```python
from build123d import *

# Parameters (mm, degrees)
SKETCH1_W           = 14
SKETCH1_H           = 80
BOSS_EXTRUDE1_DEPTH = 2
SKETCH2_W           = 14
SKETCH2_H           = 80
SKETCH2_W_2         = 10
SKETCH2_H_2         = 75
BOSS_EXTRUDE2_DEPTH = 10
SKETCH3_W           = 1
SKETCH3_H           = 3
CUT_EXTRUDE1_DEPTH  = 10
CUT_EXTRUDE2_DEPTH  = 14
SKETCH5_W           = 15
SKETCH5_H           = 80
BOSS_EXTRUDE3_DEPTH = 2
SKETCH6_W           = 15
SKETCH6_H           = 3
BOSS_EXTRUDE4_DEPTH = 12
SKETCH7_R           = 4.5
CUT_EXTRUDE3_DEPTH  = 80
SKETCH8_W           = 2
SKETCH8_H           = 74
BOSS_EXTRUDE5_DEPTH = 12


with BuildPart() as part:
    # Sketch1 → Boss-Extrude1 (new body)
    with BuildSketch(Plane(origin=(0, 0, 0), x_dir=(1, 0, 0), z_dir=(0, 1, 0))):
        Rectangle(SKETCH1_W, SKETCH1_H)
    extrude(amount=BOSS_EXTRUDE1_DEPTH)

    # Sketch2 → Boss-Extrude2 (add)
    with BuildSketch(Plane(origin=(0, 2, 0), x_dir=(1, 0, 0), z_dir=(0, 1, 0))):
        Rectangle(SKETCH2_W, SKETCH2_H)
        Rectangle(SKETCH2_W_2, SKETCH2_H_2, mode=Mode.SUBTRACT)
    extrude(amount=BOSS_EXTRUDE2_DEPTH)

    # Sketch3 → Cut-Extrude1 (cut)
    with BuildSketch(Plane(origin=(0, 12, 0), x_dir=(1, 0, 0), z_dir=(0, 1, 0))):
        with Locations((-5.5, -32)):
            Rectangle(SKETCH3_W, SKETCH3_H)
        with Locations((5.5, -32)):
            Rectangle(SKETCH3_W, SKETCH3_H)
        with Locations((5.5, 32)):
            Rectangle(SKETCH3_W, SKETCH3_H)
        with Locations((-5.5, 32)):
            Rectangle(SKETCH3_W, SKETCH3_H)
    extrude(amount=-CUT_EXTRUDE1_DEPTH, mode=Mode.SUBTRACT)

    # Sketch4 → Cut-Extrude2 (cut)
    with BuildSketch(Plane(origin=(7, 0, 0), x_dir=(0, 0, -1), z_dir=(1, 0, 0))):
        with BuildLine():
            ThreePointArc((-37.5, 5), (-32.5, 10), (-27.5, 5))
            Line((-27.5, 5), (-27.5, 2))
            Line((-27.5, 2), (-32.5, 2))
            Line((-32.5, 2), (-37.5, 2))
            Line((-37.5, 2), (-37.5, 5))
        make_face()
        with BuildLine():
            ThreePointArc((27.5, 5), (32.5, 10), (37.5, 5))
            Line((37.5, 5), (37.5, 2))
            Line((37.5, 2), (32.5, 2))
            Line((32.5, 2), (27.5, 2))
            Line((27.5, 2), (27.5, 5))
        make_face()
    extrude(amount=-CUT_EXTRUDE2_DEPTH, mode=Mode.SUBTRACT)

    # Sketch5 → Boss-Extrude3 (add)
    with BuildSketch(Plane(origin=(0, 0, 0), x_dir=(1, 0, 0), z_dir=(0, 1, 0))):
        with Locations((14.5, 0)):
            Rectangle(SKETCH5_W, SKETCH5_H)
    extrude(amount=BOSS_EXTRUDE3_DEPTH)

    # Sketch6 → Boss-Extrude4 (add)
    with BuildSketch(Plane(origin=(0, 2, 0), x_dir=(1, 0, 0), z_dir=(0, 1, 0))):
        with Locations((14.5, -38.5)):
            Rectangle(SKETCH6_W, SKETCH6_H)
        with Locations((14.5, 38.5)):
            Rectangle(SKETCH6_W, SKETCH6_H)
    extrude(amount=BOSS_EXTRUDE4_DEPTH)

    # Sketch7 → Cut-Extrude3 (cut)
    with BuildSketch(Plane.XY.offset(40)):
        with Locations((14, 8)):
            Circle(SKETCH7_R)
    extrude(amount=-CUT_EXTRUDE3_DEPTH, mode=Mode.SUBTRACT)

    # Sketch8 → Boss-Extrude5 (add)
    with BuildSketch(Plane(origin=(0, 2, 0), x_dir=(1, 0, 0), z_dir=(0, 1, 0))):
        with Locations((21, 0)):
            Rectangle(SKETCH8_W, SKETCH8_H)
    extrude(amount=BOSS_EXTRUDE5_DEPTH)


solid = part.part
```
The listing builds one solid part. Answer for the finished solid, in the listing's coordinates (mm). A direction names the side the tool comes from. Coordinates: 2 decimals unless noted, no trailing zeros. Write each loop counter-clockwise with the first axis right and the second up, starting at its lowest first coordinate (ties: lowest second). Pieces come first, ordered by that corner, then holes. Notation, with made-up numbers: (0, -5) - (26, -5) arc R9 ccw to (26, 10) - close; hole circle Ø9 at (10.25, 59). An arc over 180 degrees is marked (long way). Return JSON: item names as keys, results as strings. Group by question number.
Q1. The part is cut by section C-C on z = 17. Write down the section's boundary in (x, y), and give its area (3 significant figures).
Q2. Flat-ended cylindrical pins translate along their axes: pin 1 Ø2 at (x, z) = (13.5, 0.5) entering from +Y; pin 2 Ø4 at (y, z) = (3, 30) entering from -X; pin 3 Ø5.5 at (x, y) = (14, 8) entering from +Z; pin 4 Ø15.5 at (x, z) = (-1, -11) entering from +Y. Find the tip coordinate at first contact, or state that the pin passes through.
Q3. Find the intervals of material crossed by line 1 along X through (y, z) = (11, -1); line 2 along Z through (x, y) = (15.75, 12.5); line 3 along Z through (x, y) = (-2.5, 5.5), in increasing order. Write a range as [from, to].
Q4. The part is cut by section B-B on z = 32.5. Write down the section's boundary in (x, y), and give its area (3 significant figures).
Q5. For a pull along X with two mould halves and no side action, classify faces 1 (the flat face through (21, 14, 3)), 2 (the flat face through (5, 7, 0)) as +X half, -X half, draft (parallel to the pull), parting line (faces both ways), or undercut.
Q6. The part is cut by section A-A on x = 14. Write down the section's boundary in (y, z), and give its area (3 significant figures).
Q7. Which of the six approach directions +Z, -Z, +X, -X, +Y, -Y give full straight-line access (tool end or side, diameter ignored) to faces 3 (the flat face through (6, 3, -27.5)), 4 (the flat face through (7, 0, -1)), 5 (the flat face through (-5, 10, -36))?
Q8. The part is cut by section D-D on y = 13.25. Write down the section's boundary in (x, z).
Evaluation:
{
 "1": {"outline": "(-7, 0) - (22, 0) - (22, 14) - (20, 14) - (20, 2) - (7, 2) - (7, 12) - (5, 12) - (5, 2) - (-5, 2) - (-5, 12) - (-7, 12) - close", "area": "122 mm2"},
 "2": {"pin 1": "stops at y = 2", "pin 2": "stops at x = -7", "pin 3": "passes through", "pin 4": "stops at y = 12"},
 "3": {"line 1": "x = [-7, -5], [5, 7], [20, 22]", "line 2": "z = [-40, -37], [37, 40]", "line 3": "z = [-40, -37.5], [37.5, 40]"},
 "4": {"outline": "(-7, 0) - (22, 0) - (22, 14) - (20, 14) - (20, 2) - (-7, 2) - close; (-7, 10) - (-6, 10) - (-6, 12) - (-7, 12) - close; (6, 10) - (7, 10) - (7, 12) - (6, 12) - close", "area": "86.0 mm2"},
 "5": {"face 1": "draft", "face 2": "undercut"},
 "6": {"outline": "(0, -40) - (3.5, -40) - (3.5, -37) - (2, -37) - (2, 37) - (3.5, 37) - (3.5, 40) - (0, 40) - close; (12.5, -40) - (14, -40) - (14, -37) - (12.5, -37) - close; (12.5, 37) - (14, 37) - (14, 40) - (12.5, 40) - close", "area": "178 mm2"},
 "7": {"face 3": "-X", "face 4": "+Z, -Z, +X, -X, -Y", "face 5": "+Y"},
 "8": {"outline": "(7, -40) - (22, -40) - (22, 40) - (7, 40) - (7, 37) - (20, 37) - (20, -37) - (7, -37) - close"}
}
